Part model, mm, in its own coordinate system. Give positions to 0.01 mm unless a question says otherwise; leave off trailing zeros. Write each loop counter-clockwise with the first axis right and the second up, starting at its lowest first coordinate (ties: lowest second). Pieces come first, ordered by that corner, then holes. Notation, with made-up numbers: M -21,50.5 L -13,50.5 A19 cw -13,73.5 Z; hole C 7,51 d8. An arc over 180 degrees is marked long. Use CSV: the item, a comma, the result in double quotes. Start each with the question number.
1. Band-saw the part on B-B, the plane x = 15.5. List the corners of the cut face in (y, z).
2. Drop flat-ended pins along their axis: pin 1 Ø3 at (x, z) = (9.5, 2.5) entering from -Y; pin 2 Ø3 at (x, y) = (22, 36.5) entering from +Z; pin 3 Ø1.8 at (x, z) = (8.5, 3) entering from +Y; pin 4 Ø1.8 at (x, z) = (8, 4) entering from +Y. Give the stop position or say it passes through.
3. Drill centre lines: line 1 along Y through (x, z) = (49.5, 5.2); line 2 along Y through (x, z) = (92, 3.1) (3 decimals); line 3 along Y through (x, z) = (76, 4.6). Where is each one in solid material? Low to high. Write a range as from..to.
4. Band-saw the part on A-A, the plane y = 55.5. List the corners of the cut face in (x, z), then the cut area to 3 significant figures.
5. Band-saw the part on C-C, the plane x = 31.5. List the corners of the cut face in (y, z), then the cut area to 3 significant figures.
6. Band-saw the part on D-D, the plane y = 6.5. List the corners of the cut face in (x, z), then the cut area to 3 significant figures.
from build123d import *

# Parameters (mm, degrees)
CROQUIS1_W              = 115
CROQUIS1_H              = 80
SALIENTE_EXTRUIR1_DEPTH = 6
CROQUIS2_R              = 6
CROQUIS2_R_2            = 1.625
CROQUIS2_R_3            = 2
CORTAR_EXTRUIR1_DEPTH   = 7
REDONDEO1_R             = 12
CROQUIS3_R              = 2
CORTAR_EXTRUIR2_DEPTH   = 7


with BuildPart() as part:
    # Croquis1 → Saliente-Extruir1 (new body)
    with BuildSketch(Plane.XY):
        with Locations((57.5, 40)):
            Rectangle(CROQUIS1_W, CROQUIS1_H)
    extrude(amount=SALIENTE_EXTRUIR1_DEPTH)

    # Croquis2 → Cortar-Extruir1 (cut, through all)
    with BuildSketch(Plane(origin=(0, 0, 0), x_dir=(-1, 0, 0), z_dir=(0, 0, -1))):
        with Locations((-92, 40)):
            Circle(CROQUIS2_R)
        with Locations((-92, 21.75)):
            Circle(CROQUIS2_R_2)
        with Locations((-92, 58.25)):
            Circle(CROQUIS2_R_2)
        with Locations((-76, 20)):
            Circle(CROQUIS2_R_3)
        with Locations((-76, 60)):
            Circle(CROQUIS2_R_3)
        with BuildLine():
            Line((-29, 28.9), (-35, 28.9))
            ThreePointArc((-35, 28.9), (-46.1, 40), (-35, 51.1))
            Line((-35, 51.1), (-29, 51.1))
            ThreePointArc((-29, 51.1), (-17.9, 40), (-29, 28.9))
        make_face()
        with BuildLine():
            Line((-13.5, 22.85), (-19.5, 22.85))
            ThreePointArc((-19.5, 22.85), (-21.15, 24.5), (-19.5, 26.15))
            Line((-19.5, 26.15), (-13.5, 26.15))
            ThreePointArc((-13.5, 26.15), (-11.85, 24.5), (-13.5, 22.85))
        make_face()
        with BuildLine():
            Line((-44.5, 53.85), (-50.5, 53.85))
            ThreePointArc((-50.5, 53.85), (-52.15, 55.5), (-50.5, 57.15))
            Line((-50.5, 57.15), (-44.5, 57.15))
            ThreePointArc((-44.5, 57.15), (-42.85, 55.5), (-44.5, 53.85))
        make_face()
        with BuildLine():
            Line((-44.5, 22.85), (-50.5, 22.85))
            ThreePointArc((-50.5, 22.85), (-52.15, 24.5), (-50.5, 26.15))
            Line((-50.5, 26.15), (-44.5, 26.15))
            ThreePointArc((-44.5, 26.15), (-42.85, 24.5), (-44.5, 22.85))
        make_face()
        with BuildLine():
            Line((-13.5, 53.85), (-19.5, 53.85))
            ThreePointArc((-19.5, 53.85), (-21.15, 55.5), (-19.5, 57.15))
            Line((-19.5, 57.15), (-13.5, 57.15))
            ThreePointArc((-13.5, 57.15), (-11.85, 55.5), (-13.5, 53.85))
        make_face()
        with BuildLine():
            Line((-52.57, 13.93), (-58.57, 13.93))
            ThreePointArc((-58.57, 13.93), (-61.07, 16.43), (-58.57, 18.93))
            Line((-58.57, 18.93), (-52.57, 18.93))
            ThreePointArc((-52.57, 18.93), (-50.07, 16.43), (-52.57, 13.93))
        make_face()
        with BuildLine():
            Line((-5.43, 13.93), (-11.43, 13.93))
            ThreePointArc((-11.43, 13.93), (-13.93, 16.43), (-11.43, 18.93))
            Line((-11.43, 18.93), (-5.43, 18.93))
            ThreePointArc((-5.43, 18.93), (-2.93, 16.43), (-5.43, 13.93))
        make_face()
        with BuildLine():
            Line((-52.57, 61.07), (-58.57, 61.07))
            ThreePointArc((-58.57, 61.07), (-61.07, 63.57), (-58.57, 66.07))
            Line((-58.57, 66.07), (-52.57, 66.07))
            ThreePointArc((-52.57, 66.07), (-50.07, 63.57), (-52.57, 61.07))
        make_face()
        with BuildLine():
            Line((-5.43, 61.07), (-11.43, 61.07))
            ThreePointArc((-11.43, 61.07), (-13.93, 63.57), (-11.43, 66.07))
            Line((-11.43, 66.07), (-5.43, 66.07))
            ThreePointArc((-5.43, 66.07), (-2.93, 63.57), (-5.43, 61.07))
        make_face()
    extrude(amount=-CORTAR_EXTRUIR1_DEPTH, mode=Mode.SUBTRACT)

    # Redondeo1
    redondeo1_edges = [part.edges().sort_by_distance(p)[0] for p in [
        (0, 80, 3),
        (115, 80, 3),
        (115, 0, 3),
        (0, 0, 3),
    ]]
    fillet(redondeo1_edges, radius=REDONDEO1_R)

    # Croquis3 → Cortar-Extruir2 (cut, through all)
    with BuildSketch(Plane(origin=(0, 0, 0), x_dir=(-1, 0, 0), z_dir=(0, 0, -1))):
        with Locations((-21, 6.5)):
            Circle(CROQUIS3_R)
        with Locations((-62, 6.5)):
            Circle(CROQUIS3_R)
        with Locations((-62, 73.5)):
            Circle(CROQUIS3_R)
        with Locations((-21, 73.5)):
            Circle(CROQUIS3_R)
        with Locations((-52, 6.5)):
            Circle(CROQUIS3_R)
        with Locations((-52, 73.5)):
            Circle(CROQUIS3_R)
    extrude(amount=-CORTAR_EXTRUIR2_DEPTH, mode=Mode.SUBTRACT)


solid = part.part
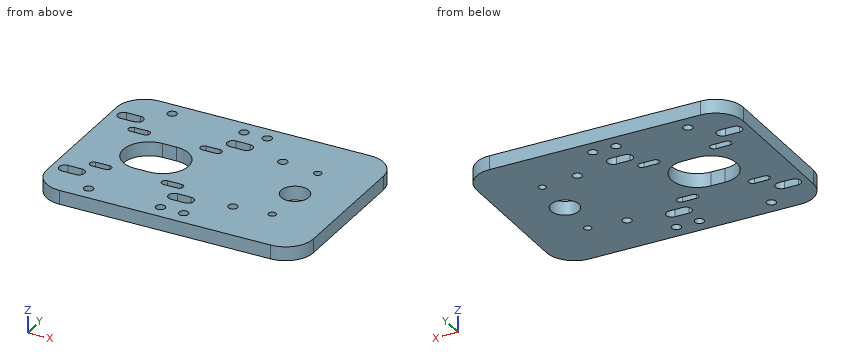
Output:
1,outline,"M 0,0 L 22.85,0 L 22.85,6 L 0,6 Z; M 26.15,0 L 53.85,0 L 53.85,6 L 26.15,6 Z; M 57.15,0 L 80,0 L 80,6 L 57.15,6 Z"
2,pin 1,"stops at y = 0.04"
2,pin 2,"passes through"
2,pin 3,"stops at y = 79.71"
2,pin 4,"stops at y = 79.59"
3,line 1,"y = 0..22.85, 26.15..53.85, 57.15..80"
3,line 2,"y = 0..20.125, 23.375..34, 46..56.625, 59.875..80"
3,line 3,"y = 0..18, 22..58, 62..80"
4,outline,"M 0,0 L 11.85,0 L 11.85,6 L 0,6 Z; M 21.15,0 L 42.85,0 L 42.85,6 L 21.15,6 Z; M 52.15,0 L 115,0 L 115,6 L 52.15,6 Z"
4,area,"578 mm²"
5,outline,"M 0,0 L 28.9,0 L 28.9,6 L 0,6 Z; M 51.1,0 L 80,0 L 80,6 L 51.1,6 Z"
5,area,"347 mm²"
6,outline,"M 1.33,0 L 19,0 L 19,6 L 1.33,6 Z; M 23,0 L 50,0 L 50,6 L 23,6 Z; M 54,0 L 60,0 L 60,6 L 54,6 Z; M 64,0 L 113.67,0 L 113.67,6 L 64,6 Z"
6,area,"602 mm²"
